Input: part model. Units: mm. Frame: model coordinates. Face numbers are marked on the shaded views. Round coordinates to 2 decimals unless told otherwise and drop trailing zeros. Loops run counter-clockwise (first coordinate to the right, second up) from the corner with the lowest first, then second, coordinate; pieces in that order, holes last. Notation, with made-up numbers: (24, 36.25) -> (75, 36.25) arc R25 ccw to (75, 74.25) -> close; hole circle Ø4 at (-11, -28.75). An arc over 180 degrees is marked (long way). Answer as a JSON object with one key per item and string values.
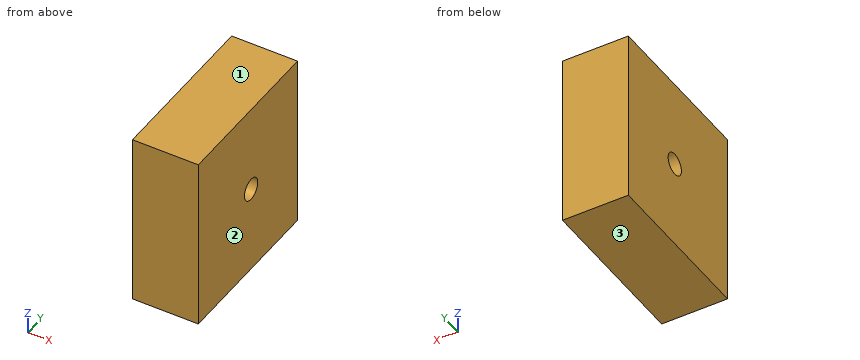
```python
from build123d import *

# Parameters (mm, degrees)
SKETCH1_W                  = 19.05
SKETCH1_H                  = 50.8
BOSS_EXTRUDE1_DEPTH        = 47.498
F_1_4_0_2500_DOWEL_HOLE1_D = 6.35


with BuildPart() as part:
    # Sketch1 → Boss-Extrude1 (new body)
    with BuildSketch(Plane(origin=(0, 0, 0), x_dir=(1, 0, 0), z_dir=(0, 1, 0))):
        Rectangle(SKETCH1_W, SKETCH1_H)
    extrude(amount=BOSS_EXTRUDE1_DEPTH)

    # 1/4 (0.2500) Dowel Hole1 (through all)
    with Locations(Plane.ZY.offset(9.525)):
        with Locations((0, 25.273)):
            Hole(F_1_4_0_2500_DOWEL_HOLE1_D / 2)


solid = part.part
```
1) Section A-A, the plane z = 0. Output: boundary loops of the cut face in (x, y) (3 decimals), plus the area to 3 significant figures.
Output:
{"outline": "(-9.525, 0) -> (9.525, 0) -> (9.525, 22.098) -> (-9.525, 22.098) -> close; (-9.525, 28.448) -> (9.525, 28.448) -> (9.525, 47.498) -> (-9.525, 47.498) -> close", "area": "784 mm^2"}
2) Contact query for a flat-ended pin moving along its axis: P1, Ø5, axis at y = 25.273, z = 0, coming from the -X side. Output: stop coordinate, or through.
Output:
{"P1": "passes through"}
3) Ray query, probe 1 along Y at (x, z) = (-2.75, 0); probe 2 along Z at (x, y) = (6.75, 24); probe 3 along Z at (x, y) = (0.75, 23.5). Return the intervals inside material, ascending.
Output:
{"probe 1": "y = 0 to 22.1, 28.45 to 47.5", "probe 2": "z = -25.4 to -2.91, 2.91 to 25.4", "probe 3": "z = -25.4 to -2.63, 2.63 to 25.4"}
4) Draft query along Z for the marked faces 1, 2 and 3. Return one class per face: +Z half, -Z half, draft (parallel to the pull), parting line (faces both ways), or undercut.
Output:
{"face 1": "+Z half", "face 2": "draft", "face 3": "-Z half"}
5) Section B-B, the plane y = 26. Output: boundary loops of the cut face in (x, z) (3 decimals), plus the area to 3 significant figures.
Output:
{"outline": "(-9.525, -25.4) -> (9.525, -25.4) -> (9.525, -3.091) -> (-9.525, -3.091) -> close; (-9.525, 3.091) -> (9.525, 3.091) -> (9.525, 25.4) -> (-9.525, 25.4) -> close", "area": "850 mm^2"}
